Here's the drawing with two shaded views (mm, measured from the low corner). I have some questions. Round coordinates to 2 decimals unless told otherwise and drop trailing zeros. Loops run counter-clockwise (first coordinate to the right, second up) from the corner with the lowest first, then second, coordinate; pieces in that order, holes last.
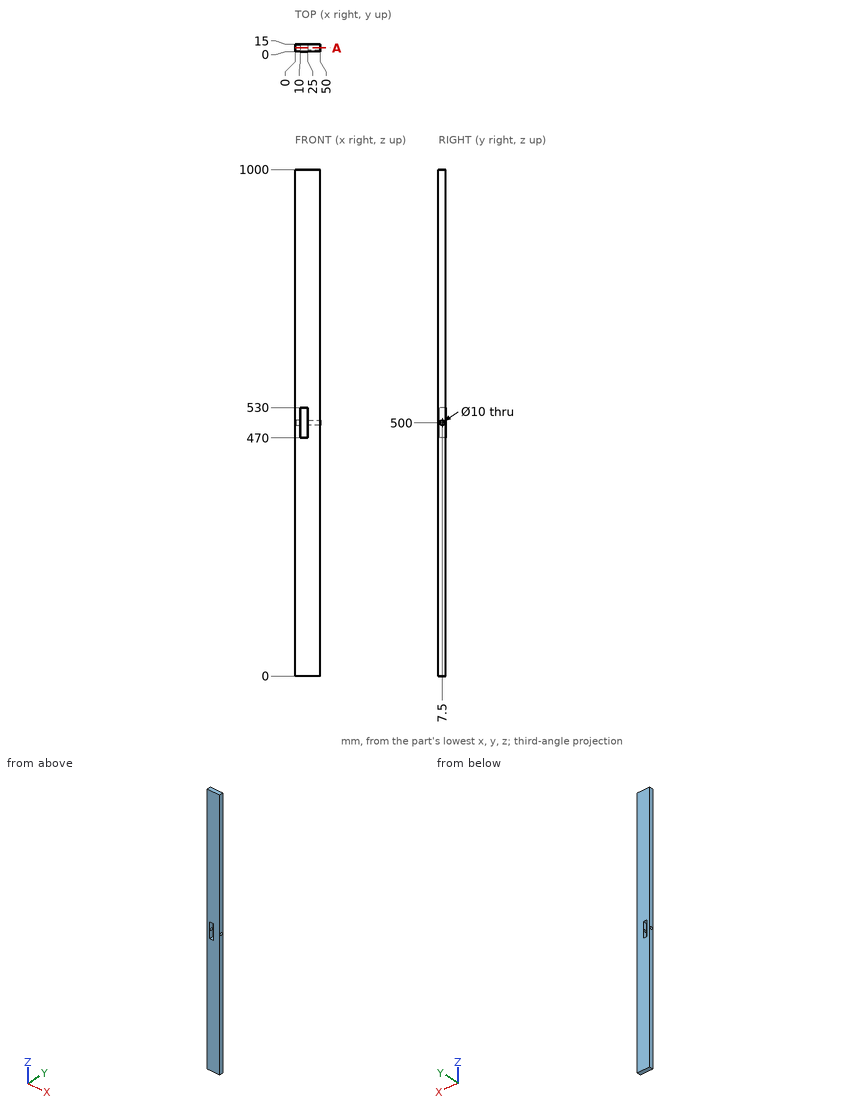
(1) If I drill on line 1 (Y direction, x = 5.5, z = 500); line 2 (Z direction, x = 5, y = 7.5); line 3 (Z direction, x = 29, y = 9.5), over which ranges is the centre line in solid material (lowest first)?
Worked answers:
line 1: y = 0 to 2.5, 12.5 to 15
line 2: z = 0 to 495, 505 to 1000
line 3: z = 0 to 495.42, 504.58 to 1000
(2) If we section it at A-A, the plane y = 7.5: List the corners of the cut face in (x, z) for me.
Worked answers:
outline: (0, 0) - (50, 0) - (50, 495) - (25, 495) - (25, 470) - (10, 470) - (10, 495) - (0, 495) - close; (0, 505) - (10, 505) - (10, 530) - (25, 530) - (25, 505) - (50, 505) - (50, 1000) - (0, 1000) - close
(3) Will these pins go through, and if not, where does the flat tip stop? P1, Ø4, axis at y = 10, z = 604, coming from the -X side; P2, Ø9, axis at y = 7.5, z = 500, coming from the -X side.
Worked answers:
P1: stops at x = 0
P2: passes through
